Autodesk Inventor part; units mm, degrees
ref_plane "YZ Plane" through (0, 0, 0) normal (1, 0, 0) x (0, 1, 0)
ref_plane "XZ Plane" through (0, 0, 0) normal (0, 1, 0) x (-1, 0, 0)
ref_plane "XY Plane" through (0, 0, 0) normal (0, 0, 1) x (1, 0, 0)
sketch "Esquisse1" plane through (0, 0, 0) normal (0, 0, 1) x (1, 0, 0)
  line L0 (0, 0) -> (-20, 34.641)
  line L1 (-20, 34.641) -> (-20, 0)
  line L2 (-20, 0) -> (0, 0)
  line L3 (-20, 34.641) -> (0, 34.641)
  line L4 (0, 34.641) -> (0, 0)
  circle A0 centre (-5, 29.641) radius 5
  circle A1 centre (-5, 29.641) radius 1.55
  line L5 (-7.0785, 26.041) -> (-9.1569, 29.641)
  line L6 (-9.1569, 29.641) -> (-7.0785, 33.241)
  line L7 (-7.0785, 33.241) -> (-2.9215, 33.241)
  line L8 (-2.9215, 33.241) -> (-0.8431, 29.641)
  line L9 (-0.8431, 29.641) -> (-2.9215, 26.041)
  line L10 (-2.9215, 26.041) -> (-7.0785, 26.041)
  line L11 (-20, 0) -> (-20, -7)
  line L12 (-20, -7) -> (0, -7)
  line L13 (0, -7) -> (0, 0)
  line L14 (-20, -3.5) -> (0, -3.5)
  circle A2 centre (-16.5, -3.5) radius 3.5
  circle A3 centre (-3.5, -3.5) radius 3.5
  circle A4 centre (-16.5, -3.5) radius 1.55
  circle A5 centre (-3.5, -3.5) radius 1.55
  point P0 (-16.5, -7)
  point P1 (-3.5, -7)
  point P2 (0, 29.641)
  point P3 (-5, 34.641)
  dimension "d0" = 60
  dimension "d1" = 20
  dimension "d5" = 7
  dimension "d6" = 3.1
  dimension "d7" = 10
  dimension "d8" = 7.2
  dimension "d9" = 3.1
extrude "Extrusion1" add sketch "Esquisse1" along normal blind 100 contours L2 L1 L0
extrude "Extrusion2" add sketch "Esquisse1" against normal blind 6 contours L2 L1 L0 | L13 A3 L2 | L0 L3 A0 L4 | A3 L14 A2 L2 | A3 L14 A5 | A0 | A3 L14 A5 | L2 A2 L11 | A2 L14 A4 | A3 L12 A2 L14 | L14 A4 A2 | L5 L6 L7 L8 L9 L10
extrude "Extrusion3" cut sketch "Esquisse1" against normal blind 3 contours L5 L6 L7 L8 L9 L10
sketch "Esquisse2" plane through (0, 0, 0) normal (1, 0, 0) x (0, 0, -1)
  line L0 (-100, 34.641) -> (-100, 0)
  line L1 (-100, 34.641) -> (-80, 0)
  line L2 (0, 0) -> (-100, 0)
  line L3 (-80, 0) -> (-100, 0)
  line L4 (-100, 0) -> (-100, 34.641)
  dimension "d16" = 30
extrude "Extrusion4" cut sketch "Esquisse2" against normal through all
properties part number "Doigt droit"
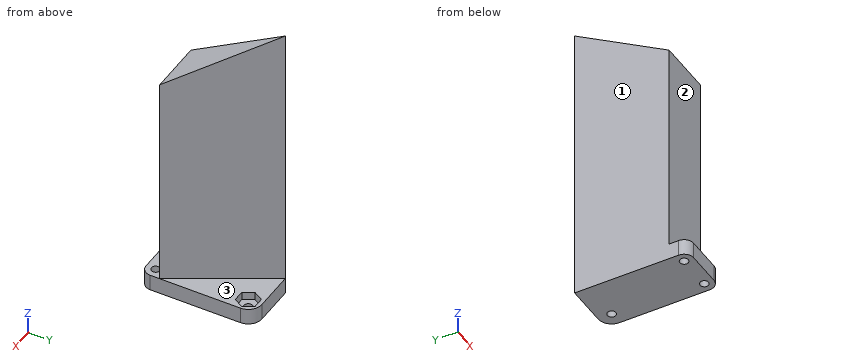
Geometry: final body of the model. Coordinates: model frame, mm. Face numbers are marked on the shaded views. A direction names the side the tool comes from. Give positions to 0.01 mm unless a question says otherwise; leave off trailing zeros. Write each loop counter-clockwise with the first axis right and the second up, starting at its lowest first coordinate (ties: lowest second). Pieces come first, ordered by that corner, then holes.
1. Line query: probe 1 along X at (y, z) = (-3.5, -1.8); probe 2 along Y at (x, z) = (-16.5, -4.4); probe 3 along Z at (x, y) = (-9.25, 18.5). Output: solid intervals per line, ascending.
2. Section query C-C, the plane y = 19. Return loops of the section in (x, z).
3. Section query B-B, the plane z = 33. Return loops of the section in (x, y).
4. Pin query (flat end, axial travel): P1, Ø10, axis at y = 10.5, z = 42.5, coming from the +X side; P2, Ø5, axis at y = 29.5, z = 86.5, coming from the +X side; P3, Ø12, axis at x = -13, z = 79, coming from the -Y side. Return the tip coordinate at first contact, or that it passes through.
5. Section query D-D, the plane y = 9. Return loops of the section in (x, z).
6. Section query A-A, the plane x = -10.75. Return loops of the section in (y, z), then the cut area to 3 significant figures.
7. Reachability of the marked faces 1, 2 and 3 from +Z, -Z, +X, -X, +Y, -Y: full face, straight path, thin tool, end or side. Return the list, or none.
Computed:
1. probe 1: x = -20 to -18.05, -14.95 to -5.05, -1.95 to 0
1. probe 2: y = -7 to -5.05, -1.95 to 34.64
1. probe 3: z = -6 to 0
2. outline: (-20, -6) - (0, -6) - (0, 0) - (-10.97, 0) - (-10.97, 90.97) - (-20, 90.97) - close
3. outline: (-20, 0) - (0, 0) - (-20, 34.64) - close
4. P1: stops at x = -3.18
4. P2: stops at x = -15.59
4. P3: stops at y = 0
5. outline: (-20, -6) - (0, -6) - (0, 0) - (-5.2, 0) - (-5.2, 85.2) - (-20, 85.2) - close
6. outline: (-7, -6) - (34.64, -6) - (34.64, 0) - (18.62, 0) - (18.62, 90.75) - (0, 80) - (0, 0) - (-7, 0) - close
6. area: 1,840 mm2
7. face 1: +Z, -Z, -X, +Y, -Y
7. face 2: +Z, +X, -X, -Y
7. face 3: +Z, +X, +Y
